from build123d import *

# Parameters (mm, degrees)
SKETCH1_W           = 35
SKETCH1_H           = 18
SKETCH1_R           = 1.5
BOSS_EXTRUDE1_DEPTH = 9
CUT_EXTRUDE1_REACH  = 28.669
SKETCH2_R           = 7.5


with BuildPart() as part:
    # Sketch1 → Boss-Extrude1 (new body)
    with BuildSketch(Plane(origin=(0, 0, 0), x_dir=(1, 0, 0), z_dir=(0, 1, 0))):
        Rectangle(SKETCH1_W, SKETCH1_H)
        with Locations(Location((-12.5, 0, 0), (0, 0, 270))):
            Circle(SKETCH1_R, mode=Mode.SUBTRACT)
        with Locations(Location((12.5, 0, 0), (0, 0, 90))):
            Circle(SKETCH1_R, mode=Mode.SUBTRACT)
    extrude(amount=BOSS_EXTRUDE1_DEPTH)

    # Sketch2 → Cut-Extrude1 (cut, up to next)
    with BuildSketch(Plane.XY.offset(9), mode=Mode.PRIVATE) as cut_extrude1_sk1:
        with Locations((0, 9)):
            Circle(SKETCH2_R)
    cut_extrude1_tool1 = extrude(cut_extrude1_sk1.sketch, amount=-CUT_EXTRUDE1_REACH, mode=Mode.PRIVATE) & part.part
    add(cut_extrude1_tool1.solids().sort_by_distance((0, 9, 9))[0], mode=Mode.SUBTRACT)


solid = part.part
CAD build for the part. Positions are in the model's coordinates, mm. Round coordinates to 2 decimals unless told otherwise and drop trailing zeros. Write each loop counter-clockwise with the first axis right and the second up, starting at its lowest first coordinate (ties: lowest second). Pieces come first, ordered by that corner, then holes. Notation, with made-up numbers: M -39.5,18 L -22.5,18 A22 cw -22.5,37 Z; hole C 88.25,59 d9. An arc over 180 degrees is marked long. Use a Markdown table: item, result. Add a question column.
1. Pull direction X, two halves, no side cores. Call faces 1 (the face through (0, 1, -9)), 2 (the face through (17.5, 4, 0)), 3 (the face through (-0.16, 1.5, 0.13)), 4 (the face through (-12.05, 4.44, 1.43)): released by +X, released by -X, zero draft, split by the parting line, or undercut.
2. Slice it at D-D on z = 5. Give the cut face in (x, y), then the cut area to 3 significant figures.
3. Drill centre lines: probe 1 along Z at (x, y) = (12.5, 4.25); probe 2 along X at (y, z) = (6.75, 0); probe 3 along X at (y, z) = (0.75, -0.25). Where is each one in solid material? Low to high.
4. Slice it at A-A on z = 0. Give the cut face in (x, y).
5. Slice it at C-C on x = 12.5. Give the cut face in (y, z).
6. Slice it at B-B on y = 7. Give the cut face in (x, z), then the cut area to 3 significant figures.
7. Flat gauge pin, fed straight in: P1, Ø1, axis at x = -8.5, z = 1.5, coming from the -Y side. Where does the tip first touch, or does it go through?
Reply:
| question | item | result |
|---|---|---|
| 1 | face 1 | zero draft |
| 1 | face 2 | released by +X |
| 1 | face 3 | undercut |
| 1 | face 4 | undercut |
| 2 | outline | M -17.5,0 L 17.5,0 L 17.5,9 L 7.5,9 A7.5 cw -7.5,9 L -17.5,9 Z |
| 2 | area | 227 mm^2 |
| 3 | probe 1 | z = -9 to -1.5, 1.5 to 9 |
| 3 | probe 2 | x = -17.5 to -14, -11 to -7.15, 7.15 to 11, 14 to 17.5 |
| 3 | probe 3 | x = -17.5 to -13.98, -11.02 to 11.02, 13.98 to 17.5 |
| 4 | outline | M -17.5,0 L -14,0 L -14,9 L -17.5,9 Z; M -11,0 L 11,0 L 11,9 L 7.5,9 A7.5 cw -7.5,9 L -11,9 Z; M 14,0 L 17.5,0 L 17.5,9 L 14,9 Z |
| 5 | outline | M 0,-9 L 9,-9 L 9,-1.5 L 0,-1.5 Z; M 0,1.5 L 9,1.5 L 9,9 L 0,9 Z |
| 6 | outline | M -17.5,-9 L -7.23,-9 L -7.23,9 L -17.5,9 Z; M 7.23,-9 L 17.5,-9 L 17.5,9 L 7.23,9 Z; hole C -12.5,0 d3; hole C 12.5,0 d3 |
| 6 | area | 356 mm^2 |
| 7 | P1 | stops at y = 0 |
